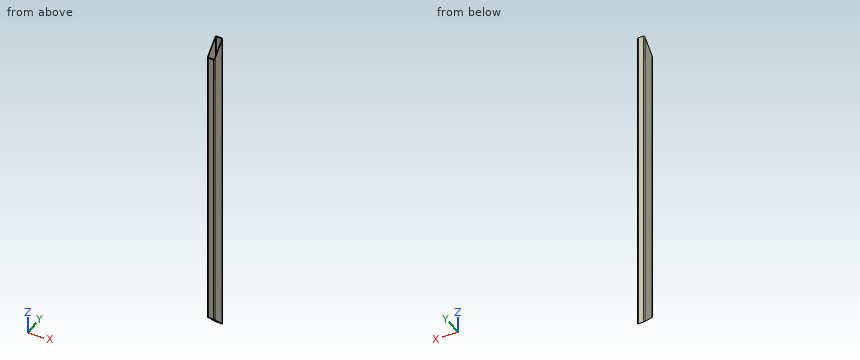
Autodesk Inventor part; units mm, degrees
ref_plane "Start Plane" through (0, 0, 0) normal (0, 0, 1) x (1, 0, 0)
ref_plane "End Plane" through (0, 0, 1700) normal (0, 0, 1) x (1, 0, 0)
ref_plane "Work Plane4" through (0, 40, 1700) normal (0, -0.7071, 0.7071) x (1, 0, 0)
ref_plane "Start Plane" through (0, 0, 0) normal (0, 0, 1) x (1, 0, 0)
ref_plane "End Plane" through (0, 0, 1700) normal (0, 0, 1) x (1, 0, 0)
sketch "Sketch" plane through (0, 0, 0) normal (0, 0, 1) x (1, 0, 0)
  line L0 (-20, -34) -> (-20, 34)
  line L1 (-14, 40) -> (14, 40)
  line L2 (20, 34) -> (20, -34)
  line L3 (14, -40) -> (-14, -40)
  arc A0 (-20, -34) -> (-14, -40) centre (-14, -34) ccw
  arc A1 (20, 34) -> (14, 40) centre (14, 34) ccw
  arc A2 (-14, 40) -> (-20, 34) centre (-14, 34) ccw
  arc A3 (14, -40) -> (20, -34) centre (14, -34) ccw
  arc A4 (-14, 37) -> (-17, 34) centre (-14, 34) ccw
  line L4 (-14, 37) -> (14, 37)
  arc A5 (17, 34) -> (14, 37) centre (14, 34) ccw
  line L5 (17, 34) -> (17, -34)
  arc A6 (14, -37) -> (17, -34) centre (14, -34) ccw
  line L6 (14, -37) -> (-14, -37)
  arc A7 (-17, -34) -> (-14, -37) centre (-14, -34) ccw
  line L7 (-17, -34) -> (-17, 34)
  line L8 (0, 57.7397) -> (0, -57.7397) construction
  line L9 (-29.7397, 0) -> (29.7397, 0) construction
  dimension "d7" = 6
  dimension "d9" = 40
  dimension "d11" = 80
  dimension "d12" = 3
  dimension "d15" = 20
  dimension "d16" = 40
extrude "Body" add sketch "Sketch" along normal up to surface (1700 mm away) from surface at 0
sketch "Sketch3" plane through (0, 0, 0) normal (0, 0, 1) x (1, 0, 0)
  line L0 (0, 0) -> (10, 0)
ref_plane "Work Plane3" through (0, 0, 0) normal (0, -1, 0) x (1, 0, 0)
ref_plane "Work Plane4" through (0, 40, 1700) normal (0, -0.7071, 0.7071) x (1, 0, 0)
split "Split1" plane through (0, 40, 1700) removes the side toward (0, -0.7071, 0.7071)
ref_plane "Work Plane5" through (0, 40, 0) normal (0, -0.7071, -0.7071) x (1, 0, 0)
split "Split2" plane through (0, 40, 0) removes the side toward (0, -0.7071, -0.7071)
sketch "Sketch4" plane through (0, 0, 0) normal (0, -1, 0) x (1, 0, 0)
  line L0 (-2, 0) -> (12, 0)
  line L1 (-2, 1700) -> (12, 1700)
  dimension "d18" = 1700
equation "\"d7\" = G_IR"
equation "\"d9\" = G_W"
equation "\"d11\" = G_H"
equation "\"d12\" = G_T"
equation "\"d15\" = 0.5 * d9"
equation "\"d16\" = 0.5 * d11"
equation "\"d3\" = G_L"
equation "\"G_W\" = 40"
equation "\"G_H\" = 80"
equation "\"G_T\" = 3"
equation "\"G_IR\" = 6"
equation "\"G_L\" = d18"
equation "\"G_OFFSET_START\" = 0"
equation "\"G_OFFSET_END\" = 0"
properties part number "ISO 10799-2 - 80x40x3 - 1700" material "Stainless Steel"
Verification items for the finished model (mm, model axes). Give positions to 0.01 mm unless a question says otherwise; leave off trailing zeros. Write each loop counter-clockwise with the first axis right and the second up, starting at its lowest first coordinate (ties: lowest second). Pieces come first, ordered by that corner, then holes. Notation, with made-up numbers: M 54,70.5 L 72,70.5 A24 cw 72,88.5 Z; hole C 58.5,75.5 d9. An arc over 180 degrees is marked long. One line per question, with ' | ' between items.
1) Gauge pin test, flat end, axial feed: pin 1 Ø12 at (x, y) = (-12.5, -2.5) entering from +Z. Record the tip position at first contact, or that the pin passes through.
Result:
pin 1: stops at z = 1661.47
2) Section check C-C on z = 424.5. Enter the section's corners in (x, y).
Result:
outline: M -20,-34 A6 ccw -14,-40 L 14,-40 A6 ccw 20,-34 L 20,34 A6 ccw 14,40 L -14,40 A6 ccw -20,34 Z; hole M -17,-34 A3 ccw -14,-37 L 14,-37 A3 ccw 17,-34 L 17,34 A3 ccw 14,37 L -14,37 A3 ccw -17,34 Z
3) Thickness scan on line 1 along X through (y, z) = (-7, 260.5); line 2 along Y through (x, z) = (-8, 130); line 3 along X through (y, z) = (-35, 682). Record the ranges inside material, lowest first. Write a range as [from, to].
Result:
line 1: x = [-20, -17], [17, 20] | line 2: y = [-40, -37], [37, 40] | line 3: x = [-19.92, -16.83], [16.83, 19.92]
4) Section check A-A on y = -9.5. Enter the section's corners in (x, z).
Result:
outline: M -20,49.5 L -17,49.5 L -17,1650.5 L -20,1650.5 Z; M 17,49.5 L 20,49.5 L 20,1650.5 L 17,1650.5 Z
5) Section check B-B on x = 0. Enter the section's corners in (y, z).
Result:
outline: M -40,80 L -37,77 L -37,1623 L -40,1620 Z; M 37,3 L 40,0 L 40,1700 L 37,1697 Z
